from build123d import *

# Parameters (mm, degrees)
F0_R     = 12.5
F1_DEPTH = 1
F2_W     = 2
F2_H     = 7
F3_DEPTH = 3
F4_R     = 5
F5_DEPTH = 1
F6_R     = 22.5
F7_DEPTH = 15


with BuildPart() as f1:
    # F0 (on Front) → F1 (new body)
    with BuildSketch(Plane.XZ):
        Circle(F0_R)
    extrude(amount=F1_DEPTH)

    # F2 (on face) → F3 (join)
    with BuildSketch(Plane.XZ.offset(1)):
        Rectangle(F2_W, F2_H)
    extrude(amount=F3_DEPTH)

    # F4 (on face) → F5 (join)
    with BuildSketch(Plane(origin=(0, 0, 0), x_dir=(-1, 0, 0), z_dir=(0, 1, 0))):
        Circle(F4_R)
    extrude(amount=F5_DEPTH)

    # F6 (on face) → F7 (join)
    with BuildSketch(Plane(origin=(0, 1, 0), x_dir=(-1, 0, 0), z_dir=(0, 1, 0))):
        Circle(F6_R)
    extrude(amount=F7_DEPTH)


solid = f1.part
The model under review builds one solid part; all positions refer to its coordinate system, in mm. A direction names the side the tool comes from. Round coordinates to 2 decimals unless told otherwise and drop trailing zeros. Write each loop counter-clockwise with the first axis right and the second up, starting at its lowest first coordinate (ties: lowest second). Pieces come first, ordered by that corner, then holes. Notation, with made-up numbers: M -5,6 L 4,6 A20 ccw 4,29 Z; hole C 51.25,47 d3. An arc over 180 degrees is marked long. Use a Markdown table: item, result. Add a question column.
Q1. We need section D-D, the plane y = 7. State the section outline as (x, z) points.
Q2. To check wall thickness, follow line 1 (Y direction, x = -10, z = 7); line 2 (Y direction, x = -4.5, z = -2); line 3 (Y direction, x = -17.5, z = 7). State the ranges of each line that lie inside material, in increasing order.
Q3. Machinability: for faces 1 (the face through (1, -2, 0)), 2 (the face through (0, -2, 3.5)), 3 (the face through (1.08, 0.49, -4.88)), 4 (the face through (11.923, -0.493, 3.755)), which of the approach directions +Z, -Z, +X, -X, +Y, -Y give a long, thin tool a straight path to every point of the face, cutting with its end or side? Answer none if there is none.
Q4. The part is to be moulded in two halves that separate along Y. For faces 5 (the face through (0.3, 1, 5.3)), 6 (the face through (0, -2, -3.5)), 7 (the face through (-0.2, 0, -5.4)), 8 (the face through (0, -4, 0)), say which applies: pulls with the +Y half, pulls with the -Y half, needs draft (parallel to the pull), parting line crosses it, or undercut.
Q5. We need section C-C, the plane x = 0. State the section outline as (y, z) points, plus the area to 3 significant figures.
Q6. We need section B-B, the plane z = 0. State the section outline as (x, y) points.
Q7. We need section A-A, the plane x = 11. State the section outline as (y, z) points, plus the area to 3 significant figures.
Q8. Insertion check: pin 1 (4 mm diameter, centred on x = 6.5, y = 14, fed in from +Z); pin 2 (3 mm diameter, centred on x = 0.5, y = 9, fed in from -Z); pin 3 (3.5 mm diameter, centred on y = -2.5, z = 0, fed in from -X). Each pin has a flat end and moves straight along its axis. Give the tip position at first contact, or say it passes through.
Findings below:
| question | item | result |
|---|---|---|
| 1 | outline | C 0,0 d45 |
| 2 | line 1 | y = -1 to 0, 1 to 16 |
| 2 | line 2 | y = -1 to 16 |
| 2 | line 3 | y = 1 to 16 |
| 3 | face 1 | +Z, -Z, +X, -Y |
| 3 | face 2 | +Z, +X, -X, -Y |
| 3 | face 3 | none |
| 3 | face 4 | -Y |
| 4 | face 5 | undercut |
| 4 | face 6 | needs draft |
| 4 | face 7 | undercut |
| 4 | face 8 | pulls with the -Y half |
| 5 | outline | M -4,-3.5 L -1,-3.5 L -1,-12.5 L 0,-12.5 L 0,-5 L 1,-5 L 1,-22.5 L 16,-22.5 L 16,22.5 L 1,22.5 L 1,5 L 0,5 L 0,12.5 L -1,12.5 L -1,3.5 L -4,3.5 Z |
| 5 | area | 731 mm² |
| 6 | outline | M -22.5,1 L -5,1 L -5,0 L -12.5,0 L -12.5,-1 L -1,-1 L -1,-4 L 1,-4 L 1,-1 L 12.5,-1 L 12.5,0 L 5,0 L 5,1 L 22.5,1 L 22.5,16 L -22.5,16 Z |
| 7 | outline | M -1,-5.94 L 0,-5.94 L 0,5.94 L -1,5.94 Z; M 1,-19.63 L 16,-19.63 L 16,19.63 L 1,19.63 Z |
| 7 | area | 601 mm² |
| 8 | pin 1 | stops at z = 22.05 |
| 8 | pin 2 | stops at z = -22.5 |
| 8 | pin 3 | stops at x = -12.5 |
